from build123d import *

# Parameters (mm, degrees)
F0_R     = 24.75
F0_R_2   = 22.75
F1_DEPTH = 10
F2_R     = 29
F2_R_2   = 22.75
F3_DEPTH = 2
F4_SIZE  = 1


with BuildPart() as f1:
    # F0 (on Top) → F1 (new body)
    with BuildSketch(Plane.XY):
        Circle(F0_R)
        Circle(F0_R_2, mode=Mode.SUBTRACT)
    extrude(amount=F1_DEPTH)

    # F2 (on Top) → F3 (join)
    with BuildSketch(Plane.XY):
        Circle(F2_R)
        Circle(F2_R_2, mode=Mode.SUBTRACT)
    extrude(amount=F3_DEPTH)

    # F4
    f4_edges = [f1.edges().sort_by_distance(p)[0] for p in [
        (-29, 0, 0),
        (-22.75, 0, 0),
        (-24.75, 0, 10),
    ]]
    chamfer(f4_edges, length=F4_SIZE)


solid = f1.part
Work out the finished part from the listing and answer in its coordinate system (mm). A direction names the side the tool comes from. Coordinates: 2 decimals unless noted, no trailing zeros. Loops run counter-clockwise (first coordinate to the right, second up) from the corner with the lowest first, then second, coordinate; pieces in that order, holes last. Notation, with made-up numbers: M -24,81 L 15,81 A21 cw 15,108 Z; hole C -2.75,26 d4. An arc over 180 degrees is marked long. Answer in a Markdown table with one row per item. Add a question column.
1. A tool of negligible diameter and unlimited length cuts with its end or side. For faces 4 (the cylindrical face through (13.38, -25.73, 1.49)), 5 (the flat face through (21.3, 13, 2)), from which of +Z, -Z, +X, -X, +Y, -Y can it reach the whole face along a straight path? Write none if from no direction.
2. Consider L1, parallel to Y at x = 0, z = 6.25; L2, parallel to X at y = 5, z = 3.5; L3, parallel to X at y = -12, z = 6.75. Determine where each line is inside the solid, lowest interval first.
3. Find section A-A, the plane x = 0. Write down the section's boundary in (y, z).
4. Flat-ended cylindrical pins translate along their axes: P1, Ø1.5, axis at x = -15.5, z = 6, coming from the +Y side; P2, Ø6, axis at x = 0, z = 9, coming from the -Y side; P3, Ø1, axis at y = 22.5, z = 1.5, coming from the -X side. Find the tip coordinate at first contact, or state that the pin passes through.
5. The mould has two halves that part along X. Classify faces 1 (the cylindrical face through (-18.054, -13.843, 5.437)), 2 (the cylindrical face through (-3.22, 24.54, 5.45)), 3 (the flat face through (-13, -21, 0)): pulls with the +X half, pulls with the -X half, needs draft (parallel to the pull), parting line crosses it, or undercut.
6. Find section C-C, the plane z = 6.5. Write down the section's boundary in (x, y).
Reported:
| question | item | result |
|---|---|---|
| 1 | face 4 | +Z, -Z |
| 1 | face 5 | +Z |
| 2 | L1 | y = -24.75 to -22.75, 22.75 to 24.75 |
| 2 | L2 | x = -24.24 to -22.19, 22.19 to 24.24 |
| 2 | L3 | x = -21.65 to -19.33, 19.33 to 21.65 |
| 3 | outline | M -29,1 L -28,0 L -23.75,0 L -22.75,1 L -22.75,10 L -23.75,10 L -24.75,9 L -24.75,2 L -29,2 Z; M 22.75,1 L 23.75,0 L 28,0 L 29,1 L 29,2 L 24.75,2 L 24.75,9 L 23.75,10 L 22.75,10 Z |
| 4 | P1 | stops at y = 19.87 |
| 4 | P2 | stops at y = -24.75 |
| 4 | P3 | stops at x = -18.89 |
| 5 | face 1 | undercut |
| 5 | face 2 | parting line crosses it |
| 5 | face 3 | needs draft |
| 6 | outline | C 0,0 d49.5; hole C 0,0 d45.5 |
